```python
from build123d import *

# Parameters (mm, degrees)
CUT_EXTRUDE1_DEPTH = 2


with BuildPart() as part:
    # Sketch1 → Revolve1 (revolve)
    with BuildSketch(Plane.XY):
        with BuildLine():
            Line((15.7465, 2), (0.2, 2))
            ThreePointArc((0.2, 2), (0.058578644, 2.058578644), (0, 2.2))
            Line((0, 2.2), (0, 3.5))
            Line((0, 3.5), (-3.8, 3.5))
            ThreePointArc((-3.8, 3.5), (-3.941421356, 3.441421356), (-4, 3.3))
            Line((-4, 3.3), (-4, 0))
            Line((-4, 0), (16, 0))
            Line((16, 0), (16, 1.7465))
            Line((16, 1.7465), (15.7465, 2))
        make_face()
    revolve(axis=Axis((-4, 0, 0), (1, 0, 0)))

    # Sketch2 → Cut-Extrude1 (cut)
    with BuildSketch(Plane.ZY.offset(4)):
        Polygon((1.535, 0.886232663), (0, 1.772465326), (-1.535, 0.886232663), (-1.535, -0.886232663), (0, -1.772465326), (1.535, -0.886232663), align=None)
    extrude(amount=-CUT_EXTRUDE1_DEPTH, mode=Mode.SUBTRACT)


solid = part.part
```
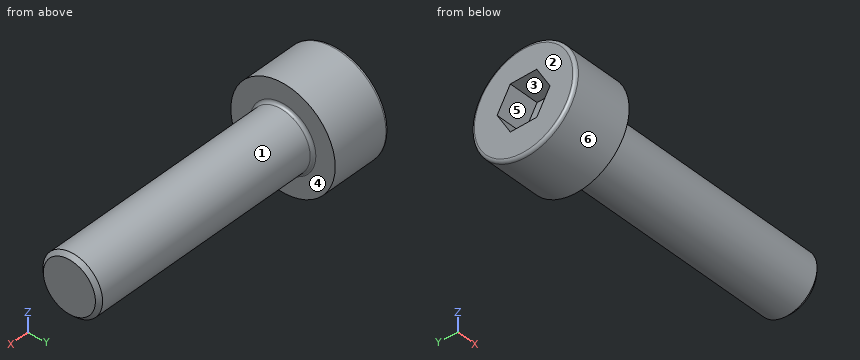
Part model, mm, in its own coordinate system. Face numbers are marked on the shaded views. A direction names the side the tool comes from. Round coordinates to 2 decimals unless told otherwise and drop trailing zeros. Loops run counter-clockwise (first coordinate to the right, second up) from the corner with the lowest first, then second, coordinate; pieces in that order, holes last.
1. Flat gauge pins, fed straight in: pin 1 (2 mm diameter, centred on x = 8, z = -2.5, fed in from -Y); pin 2 (0.9 mm diameter, centred on y = 0.5, z = 0, fed in from -X). Where does each tip first touch, or does it go through?
Solutions:
pin 1: stops at y = -1.32
pin 2: stops at x = -2
2. 3-axis set-ups, long thin cutter, end or side, ignore diameter. For the marked faces 1, 2 and 3: which of +Z, -Z, +X, -X, +Y, -Y reach the whole face in a straight line?
Solutions:
face 1: +X
face 2: +Z, -Z, -X, +Y, -Y
face 3: -X
3. Drill centre lines: line 1 along X through (y, z) = (2, -1.25); line 2 along X through (y, z) = (0.25, 0.5); line 3 along Z through (x, y) = (12, -1.5). Where is each one in solid material? Low to high.
Solutions:
line 1: x = -4 to 0
line 2: x = -2 to 16
line 3: z = -1.32 to 1.32
4. Slice it at C-C (x = 7). Give the cut face in (y, z), and give its area (3 significant figures).
Solutions:
outline: circle Ø4 at (0, 0)
area: 12.6 mm2
5. Slice it at A-A (x = -2.5). Give the cut face in (y, z) (3 decimals), and give its area (3 significant figures).
Solutions:
outline: circle Ø7 at (0, 0); hole (-1.772, 0) - (-0.886, -1.535) - (0.886, -1.535) - (1.772, 0) - (0.886, 1.535) - (-0.886, 1.535) - close
area: 30.3 mm2
6. Two-plate mould, pull along Y, no slides. Class the marked faces 4, 5 and 6: pulls with the +Y half, pulls with the -Y half, needs draft (parallel to the pull), parting line crosses it, or undercut.
Solutions:
face 4: needs draft
face 5: undercut
face 6: parting line crosses it
